```python
from build123d import *

# Parameters (mm, degrees)
SKETCH1_R           = 1.425
BOSS_EXTRUDE1_DEPTH = 5.15
FILLET1_R           = 3
BOSS_EXTRUDE2_DEPTH = 2.5
FILLET2_R           = 0.5


with BuildPart() as part:
    # Sketch1 → Boss-Extrude1 (new, symmetric)
    with BuildSketch(Plane(origin=(0, 0, 0), x_dir=(1, 0, 0), z_dir=(0, 1, 0))):
        Polygon((-8.1, 2.8), (2.8, 2.8), (2.8, -13.1), (-25, -13.1), (-25, 2.8), align=None)
        with Locations(Location((-22.2, -10.3, 0), (0, 0, 90))):
            Circle(SKETCH1_R, mode=Mode.SUBTRACT)
        with Locations(Location((0, 0, 0), (0, 0, 90))):
            Circle(SKETCH1_R, mode=Mode.SUBTRACT)
    extrude(amount=BOSS_EXTRUDE1_DEPTH, both=True)

    # Fillet1
    fillet1_edges = [part.edges().sort_by_distance(p)[0] for p in [
        (2.8, 0, -2.8),
        (2.8, 0, 13.1),
        (-25, 0, 13.1),
        (-25, 0, -2.8),
    ]]
    fillet(fillet1_edges, radius=FILLET1_R)

    # Sketch1_4 → Boss-Extrude2 (add, symmetric)
    with BuildSketch(Plane(origin=(0, 0, 0), x_dir=(1, 0, 0), z_dir=(0, 1, 0))):
        with BuildLine():
            Line((-8.35, 5.4), (-8.35, 2.8))
            Line((-8.35, 2.8), (-7.85, 2.8))
            Line((-7.85, 2.8), (-7.85, 5.9))
            Line((-7.85, 5.9), (-32.5, 5.9))
            ThreePointArc((-32.5, 5.9), (-31.763932023, 6.781966011), (-31.5, 7.9))
            Line((-31.5, 7.9), (-31.5, 11.9))
            ThreePointArc((-31.5, 11.9), (-34, 14.4), (-36.5, 11.9))
            Line((-36.5, 11.9), (-36.5, 7.9))
            ThreePointArc((-36.5, 7.9), (-35.767766953, 6.132233047), (-34, 5.4))
            Line((-34, 5.4), (-8.35, 5.4))
        make_face()
    extrude(amount=BOSS_EXTRUDE2_DEPTH, both=True)

    # Fillet2
    fillet2_edges = [part.edges().sort_by_distance(p)[0] for p in [
        (-7.85, 0, -5.9),
        (-8.35, 0, -5.4),
    ]]
    fillet(fillet2_edges, radius=FILLET2_R)


solid = part.part
```
Geometry check sheet. Reference: the model listing, model coordinates, mm. A direction names the side the tool comes from. Round coordinates to 2 decimals unless told otherwise and drop trailing zeros. Loops run counter-clockwise (first coordinate to the right, second up) from the corner with the lowest first, then second, coordinate; pieces in that order, holes last. Notation, with made-up numbers: (9.5, -30) -> (28.5, -30) arc R30 cw to (28.5, 4) -> close; hole circle Ø1 at (3, 36.5). An arc over 180 degrees is marked (long way). Use a Markdown table: item, result.
(1) Scan lines: probe 1 along Z at (x, y) = (-22.2, -0.5) (3 decimals); probe 2 along X at (y, z) = (1.75, 10.3) (3 decimals); probe 3 along X at (y, z) = (-2.75, 8.5). Record each from-to range of solid material in increasing order.
Calculated:
| item | result |
|---|---|
| probe 1 | -5.9 to -5.4, -2.793 to 8.875, 11.725 to 13.093 |
| probe 2 | -24.993 to -23.625, -20.775 to 2.793 |
| probe 3 | -25 to 2.8 |
(2) Sectioned sample at B-B (y = -3.5). Enter the section's corners in (x, z) (3 decimals).
Calculated:
| item | result |
|---|---|
| outline | (-25, 0.2) arc R3 ccw to (-22, -2.8) -> (-0.2, -2.8) arc R3 ccw to (2.8, 0.2) -> (2.8, 10.1) arc R3 ccw to (-0.2, 13.1) -> (-22, 13.1) arc R3 ccw to (-25, 10.1) -> close; hole circle Ø2.85 at (-22.2, 10.3); hole circle Ø2.85 at (0, 0) |
(3) Sectioned sample at C-C (z = -9.5). Enter the section's corners in (x, y), then the cut area to 3 significant figures.
Calculated:
| item | result |
|---|---|
| outline | (-36.5, -2.5) -> (-31.5, -2.5) -> (-31.5, 2.5) -> (-36.5, 2.5) -> close |
| area | 25.0 mm² |
(4) Go/stop test with flat-tipped pins: P1, Ø1.2, axis at y = 0, z = -10, coming from the +X side; P2, Ø2.5, axis at x = 0, z = 0, coming from the -Y side; P3, Ø2.5, axis at x = -25.5, y = -1, coming from the -Z side; P4, Ø2, axis at x = -25, z = -5, coming from the -Y side. Record where each tip stops, or that it passes through.
Calculated:
| item | result |
|---|---|
| P1 | x = -31.5 |
| P2 | through |
| P3 | z = -5.9 |
| P4 | y = -2.5 |
(5) Sectioned sample at D-D (x = -24.5). Enter the section's corners in (y, z), then the cut area to 3 significant figures.
Calculated:
| item | result |
|---|---|
| outline | (-5.15, -1.46) -> (5.15, -1.46) -> (5.15, 11.76) -> (-5.15, 11.76) -> close; (-2.5, -5.9) -> (2.5, -5.9) -> (2.5, -5.4) -> (-2.5, -5.4) -> close |
| area | 139 mm² |
(6) Mould release check, pull along Z, two halves, no side actions. Record for faces 1 (the flat face through (-32, 2.5, -9)), 2 (the flat face through (-22, 0, -5.4)), 3 (the cylindrical face through (-35.787, 0.035, -6.152)): released by +Z, released by -Z, zero draft, split by the parting line, or undercut.
Calculated:
| item | result |
|---|---|
| face 1 | zero draft |
| face 2 | undercut |
| face 3 | released by +Z |
(7) Sectioned sample at A-A (x = -17.5). Enter the section's corners in (y, z).
Calculated:
| item | result |
|---|---|
| outline | (-5.15, -2.8) -> (5.15, -2.8) -> (5.15, 13.1) -> (-5.15, 13.1) -> close; (-2.5, -5.9) -> (2.5, -5.9) -> (2.5, -5.4) -> (-2.5, -5.4) -> close |
(8) Set-up check for faces 4 (the flat face through (-7.85, 0, -4)), 5 (the flat face through (-8.35, 0, -4)), 6 (the flat face through (-32, -2.5, -9)): record each of +Z, -Z, +X, -X, +Y, -Y from which the full face is reachable in a straight line by a thin tool's end or side.
Calculated:
| item | result |
|---|---|
| face 4 | -Z, +X, +Y, -Y |
| face 5 | -X, +Y, -Y |
| face 6 | -Z, +X, -X, -Y |
